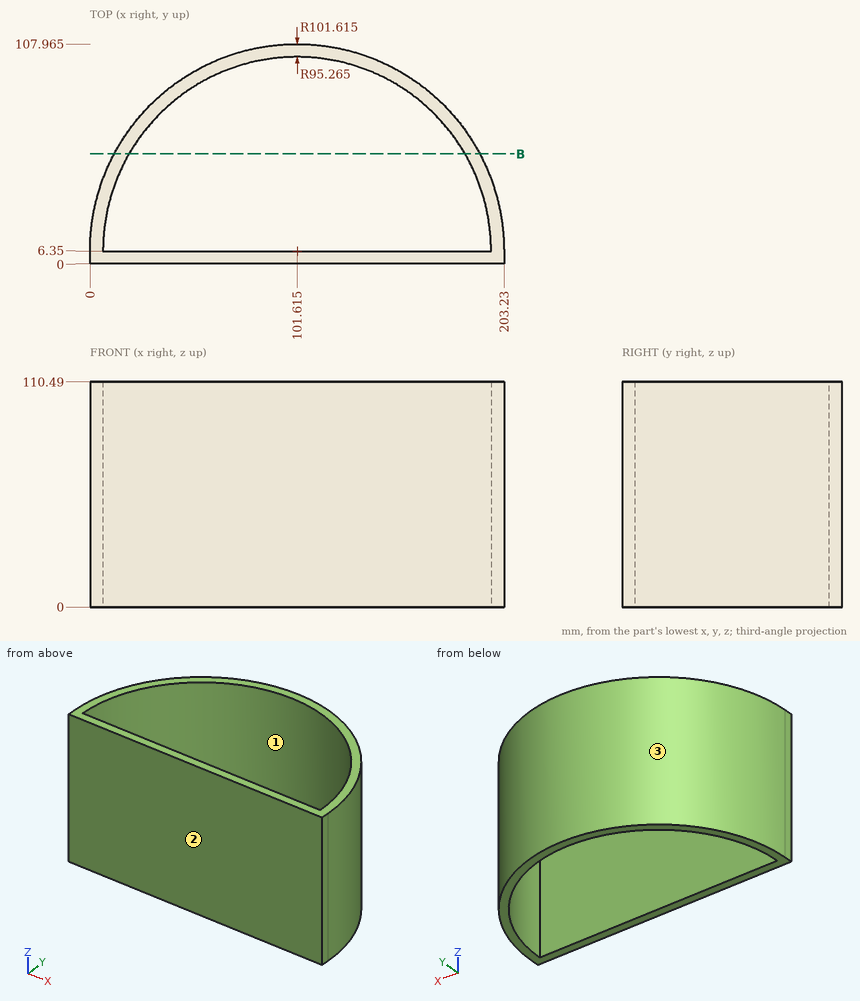
Study the drawing (mm; zero at the part's minimum x, y, z) and answer. Coordinates: 2 decimals unless noted, no trailing zeros. Write each loop counter-clockwise with the first axis right and the second up, starting at its lowest first coordinate (ties: lowest second). Pieces come first, ordered by that corner, then holes. Notation, with made-up numbers: (-37.5, 40.5) - (-7.5, 40.5) arc R29 cw to (-7.5, 66.5) - close; hole circle Ø1 at (8, -16). An arc over 180 degrees is marked (long way). Answer as a JSON object with one key per item and string values.
Q1. Consider L1, parallel to Y at x = 35, z = 18; L2, parallel to X at y = 32, z = 21; L3, parallel to Y at x = 30.5, z = 76.5. Determine where each line is inside the solid, lowest interval first. Write a range as from..to.
Results list:
{"L1": "y = 0..6.35, 74.45..83.08", "L2": "x = 3.29..9.87, 193.36..199.94", "L3": "y = 0..6.35, 69.74..78.93"}
Q2. For a pull along Y with two mould halves and no side action, classify the marked faces 1, 2 and 3 as pulls with the +Y half, pulls with the -Y half, needs draft (parallel to the pull), parting line crosses it, or undercut.
Results list:
{"face 1": "undercut", "face 2": "pulls with the -Y half", "face 3": "pulls with the +Y half"}
Q3. Find section B-B (y = 54). Write down the section's boundary in (x, z) (1 decimal).
Results list:
{"outline": "(11.9, 0) - (19.1, 0) - (19.1, 110.5) - (11.9, 110.5) - close; (184.1, 0) - (191.4, 0) - (191.4, 110.5) - (184.1, 110.5) - close"}
Q4. Given pin 1 Ø12 at (y, z) = (49, 27.5) entering from +X; pin 2 Ø6 at (y, z) = (90, 44.5) entering from -X; pin 3 Ø6 at (y, z) = (55.5, 37.5) entering from -X, each flat-ended and moving along its own axis, determine where each tip first touches the part or whether it passes through.
Results list:
{"pin 1": "stops at x = 196.39", "pin 2": "stops at x = 39.8", "pin 3": "stops at x = 11.08"}
